Autodesk Inventor part; units mm, degrees
ref_plane "YZ Plane" through (0, 0, 0) normal (1, 0, 0) x (0, 1, 0)
ref_plane "XZ Plane" through (0, 0, 0) normal (0, 1, 0) x (-1, 0, 0)
ref_plane "XY Plane" through (0, 0, 0) normal (0, 0, 1) x (1, 0, 0)
sketch "Sketch1" plane through (0, 0, 0) normal (1, 0, 0) x (0, 1, 0)
  circle A0 centre (0, 0) radius 4.435
  dimension "d0" = 8.87
extrude "Extrusion1" add sketch "Sketch1" along normal blind 280.8
sketch "Sketch2" plane through (280.8, 0, 0) normal (1, 0, 0) x (0, 0, -1)
  circle A0 centre (0, 0) radius 4.435
  line L0 (0, 0) -> (8.3226, 0)
  line L1 (0.8914, 0) -> (-7.5966, 0)
  arc A1 (-4.435, 0) -> (4.435, 0) centre (0, 0) ccw
extrude "Extrusion2" add sketch "Sketch2" along normal blind 0.01 contours A0 L1 L0 picked at (-2.4155, -1.6673)
ref_plane "Work Plane1" through (280.81, 0, 0) normal (0.3420201, 0.9396926, 0) x (0, 0, 1)
sketch "Sketch4" plane through (280.81, 0, 0) normal (0.3420201, 0.9396926, 0) x (0, 0, 1)
  line L0 (4.435, -0.0094) -> (-4.435, -0.0094)
  ellipse E0 centre (0, -0.0094) end of major axis (-4.435, -0.0094) minor radius 1.5169 (-4.435, -0.0094) -> (4.435, -0.0094) ccw
  line L1 (-4.435, 0) -> (4.435, 0)
  ellipse E1 centre (0, 0) end of major axis (-4.435, 0) minor radius 1.5169 (4.435, 0) -> (-4.435, 0) ccw
  circle A0 centre (0, 0) radius 7.85
  point P0 (0, -263.8751)
  dimension "d11" = 15.7
extrude "Extrusion4" add sketch "Sketch4" along normal blind 90 and the other way blind 90 contours E0 L0 | E1 L1 | A0
sketch "Sketch6" plane through (311.5918, 84.5723, 0) normal (0.3420201, 0.9396926, 0) x (0.9396926, -0.3420201, 0)
  circle A0 centre (0, 0) radius 7.85
  circle A1 centre (0, 0) radius 1
  circle A2 centre (0, 0) radius 2.5
  point P0 (-263.8751, 0)
  dimension "d19" = 5
extrude "Extrusion6" add sketch "Sketch6" along normal blind 12.7 contours A1 | A2
sketch "Sketch7" plane through (315.9355, 96.5064, 0) normal (0.3420201, 0.9396926, 0) x (0.9396926, -0.3420201, 0)
  circle A0 centre (0, 0) radius 2.5
  circle A1 centre (0, 0) radius 1.5
  point P0 (-263.8751, 0)
  dimension "d22" = 3
extrude "Extrusion7" add sketch "Sketch7" along normal blind 76.2 contours A1
properties part number "Piston_Model"
Work out the finished part from the listing and answer in its coordinate system (mm). A direction names the side the tool comes from. Give positions to 0.01 mm unless a question says otherwise; leave off trailing zeros. Loops run counter-clockwise (first coordinate to the right, second up) from the corner with the lowest first, then second, coordinate; pieces in that order, holes last. Notation, with made-up numbers: M 58.25,68.5 L 69.25,68.5 A17 ccw 69.25,79.5 Z; hole C -39.5,66.5 d2. An arc over 180 degrees is marked long. One line per item, written item: value. Start each with the question number.
1. Find the intervals of material crossed by probe 1 along Y at (x, z) = (80.5, -0.75); probe 2 along X at (y, z) = (-11, 7); probe 3 along Y at (x, z) = (235, -1.5), in increasing order.
2. Determine the mould class of faces 1 (the face through (0, 0, 0)), 2 (the face through (250.1, -84.6, -0.1)), 3 (the face through (315.903, 89.666, -0.958)) for opening direction Y: released by +Y, released by -Y, zero draft, split by the parting line, or undercut.
3. Which of the six approach directions +Z, -Z, +X, -X, +Y, -Y give full straight-line access (tool end or side, diameter ignored) to faces 4 (the face through (135.246, 2.046, 3.935)), 5 (the face through (311.695, 84.535, 3.379))?
4. Find section A-A (x = 113.5). Give the vertices of the cut face in (y, z) (3 decimals), and give its area (3 significant figures).
5. Each of these flat-tipped pins is pushed along its axis until it touches: P1, Ø3, axis at y = 49, z = -3, coming from the +X side; P2, Ø8, axis at y = 116.5, z = -6, coming from the -X side. Where does it stop, or does it pass through?
Reported:
1. probe 1: y = -4.37 to 4.37
1. probe 2: x = 273.03 to 280.59
1. probe 3: y = -4.17 to 4.17
2. face 1: zero draft
2. face 2: released by -Y
2. face 3: undercut
3. face 4: -X
3. face 5: none
4. outline: C 0,0 d8.87
4. area: 61.8 mm²
5. P1: stops at x = 307.13
5. P2: passes through
